Geometry: final body of the model. Coordinates: model frame, mm. A direction names the side the tool comes from. Round coordinates to 2 decimals unless told otherwise and drop trailing zeros. Order: outer loops, then holes, each group sorted by start corner. A loop starts at its lowest first (then second) coordinate and runs counter-clockwise, first axis right, second up. Notation, with made-up numbers: (21, 65.5) -> (66, 65.5) arc R18 ccw to (66, 69.5) -> close; hole circle Ø10 at (59, 82.25). An arc over 180 degrees is marked (long way). Put each result on its own line as item: value.
```python
from build123d import *

# Parameters (mm, degrees)
EXTRUDE_1_DEPTH      = 38
CUT_EXTRUDE_1_REACH  = 44.579
SKETCH_2_R           = 1.6
EXTRUDE_2_DEPTH      = 4.5
EXTRUDE_2_DEPTH_BACK = 10
SKETCH_3_R           = 1.15
CHAMFER_1_SIZE       = 0.2


with BuildPart() as part:
    # Эскиз1 → Бобышка-Вытянуть1 (new body)
    with BuildSketch(Plane.XY):
        with BuildLine():
            Line((-14.5, -3), (14.5, -3))
            Line((14.5, -3), (14.5, -1.148611647))
            ThreePointArc((14.5, -1.148611647), (14.150439729, -0.637384409), (13.547219321, -0.777637076))
            ThreePointArc((13.547219321, -0.777637076), (11.55, 0), (13.547219321, 0.777637076))
            ThreePointArc((13.547219321, 0.777637076), (13.692982689, 0.71288454), (13.839750373, 0.775327291))
            Line((13.839750373, 0.775327291), (15, 2))
            Line((15, 2), (15, 8.1))
            ThreePointArc((15, 8.1), (14.1, 9), (13.2, 8.1))
            Line((13.2, 8.1), (13.2, 2.602402736))
            ThreePointArc((13.2, 2.602402736), (11.012175957, 2.042975771), (10.05, 0))
            Line((10.05, 0), (9.55, 0))
            Line((9.55, 0), (9.55, 8.1))
            ThreePointArc((9.55, 8.1), (8.65, 9), (7.75, 8.1))
            Line((7.75, 8.1), (7.75, 0))
            Line((7.75, 0), (-7.75, 0))
            Line((-7.75, 0), (-7.75, 8.1))
            ThreePointArc((-7.75, 8.1), (-8.65, 9), (-9.55, 8.1))
            Line((-9.55, 8.1), (-9.55, 0))
            Line((-9.55, 0), (-10.05, 0))
            ThreePointArc((-10.05, 0), (-11.012175957, 2.042975771), (-13.2, 2.602402736))
            Line((-13.2, 2.602402736), (-13.2, 8.1))
            ThreePointArc((-13.2, 8.1), (-14.1, 9), (-15, 8.1))
            Line((-15, 8.1), (-15, 2))
            Line((-15, 2), (-13.839750373, 0.775327291))
            ThreePointArc((-13.839750373, 0.775327291), (-13.692982689, 0.71288454), (-13.547219321, 0.777637076))
            ThreePointArc((-13.547219321, 0.777637076), (-11.55, 0), (-13.547219321, -0.777637076))
            ThreePointArc((-13.547219321, -0.777637076), (-14.150439729, -0.637384409), (-14.5, -1.148611647))
            Line((-14.5, -1.148611647), (-14.5, -3))
        make_face()
    extrude(amount=EXTRUDE_1_DEPTH)

    # Эскиз2 → Вырез-Вытянуть1 (cut, up to next)
    with BuildSketch(Plane.XZ.offset(3), mode=Mode.PRIVATE) as cut_extrude_1_sk1:
        with Locations(Location((0, 18.3, 0), (0, 0, 270))):
            Circle(SKETCH_2_R)
    cut_extrude_1_tool1 = extrude(cut_extrude_1_sk1.sketch, amount=-CUT_EXTRUDE_1_REACH, mode=Mode.PRIVATE) & part.part
    add(cut_extrude_1_tool1.solids().sort_by_distance((0, -3, 18.3))[0], mode=Mode.SUBTRACT)

    # Эскиз3 → Бобышка-Вытянуть2 (add, two sides: drawn at the far end of the back side and taken through both)
    with BuildSketch(Plane(origin=(0, 0, 0), x_dir=(-1, 0, 0), z_dir=(0, 0, -1)).offset(-EXTRUDE_2_DEPTH_BACK)):
        with Locations((12.7, 0)):
            Circle(SKETCH_3_R)
        with Locations((-12.7, 0)):
            Circle(SKETCH_3_R)
    extrude(amount=EXTRUDE_2_DEPTH + EXTRUDE_2_DEPTH_BACK)

    # Фаска1
    chamfer_1_edges = [part.edges().sort_by_distance(p)[0] for p in [
        (-11.55, 0, -4.5),
        (13.85, 0, -4.5),
    ]]
    chamfer(chamfer_1_edges, length=CHAMFER_1_SIZE)


solid = part.part
```
1. Cut plane B-B on x = 0. Return loops of the section in (y, z), and give its area (3 significant figures).
Ans:
outline: (-3, 0) -> (0, 0) -> (0, 16.7) -> (-3, 16.7) -> close; (-3, 19.9) -> (0, 19.9) -> (0, 38) -> (-3, 38) -> close
area: 104 mm²
2. Cut plane A-A on y = 4.25. Return loops of the section in (x, z), and give its area (3 significant figures).
Ans:
outline: (-15, 0) -> (-13.2, 0) -> (-13.2, 38) -> (-15, 38) -> close; (-9.55, 0) -> (-7.75, 0) -> (-7.75, 38) -> (-9.55, 38) -> close; (7.75, 0) -> (9.55, 0) -> (9.55, 38) -> (7.75, 38) -> close; (13.2, 0) -> (15, 0) -> (15, 38) -> (13.2, 38) -> close
area: 274 mm²
3. Draft query along X for faces 1 (the face through (0, -1, 38)), 2 (the face through (-15, 5, 19)), 3 (the face through (7.75, 4, 19)), 4 (the face through (13, 0, 10)). Return one class per face: +X half, -X half, draft (parallel to the pull), parting line (faces both ways), or undercut.
Ans:
face 1: draft
face 2: -X half
face 3: undercut
face 4: undercut
4. Material intervals for probe 1 along X at (y, z) = (5, 20.5); probe 2 along Y at (x, z) = (12.7, 17.75); probe 3 along X at (y, z) = (-2.15, 18.3), sorted ascending.
Ans:
probe 1: -15 to -13.2, -9.55 to -7.75, 7.75 to 9.55, 13.2 to 15
probe 2: -3 to -1.15, 1.15 to 2.65
probe 3: -14.5 to -1.6, 1.6 to 14.5
5. Set-up query: faces 5 (the face through (13.2, 5, 19)), 6 (the face through (-14.43, 1.4, 18.73)), 7 (the face through (14.41, 1.38, 18.73)). Return all of +Z, -Z, +X, -X, +Y, -Y with unobstructed straight access to the full face (end or side cutting, diameter ignored); none if empty.
Ans:
face 5: +Z, -Z, +Y
face 6: +Z, -Z, -X
face 7: +Z, -Z, +X
6. Cut plane C-C on z = 7.5. Return loops of the section in (x, y), and give its area (3 significant figures).
Ans:
outline: (-15, 2) -> (-13.84, 0.78) arc R0.2 ccw to (-13.55, 0.78) arc R1.15 ccw to (-13.55, -0.78) arc R0.55 ccw to (-14.5, -1.15) -> (-14.5, -3) -> (14.5, -3) -> (14.5, -1.15) arc R0.55 ccw to (13.55, -0.78) arc R1.15 ccw to (13.55, 0.78) arc R0.2 ccw to (13.84, 0.78) -> (15, 2) -> (15, 8.1) arc R0.9 ccw to (13.2, 8.1) -> (13.2, 2.6) arc R2.65 ccw to (10.05, 0) -> (9.55, 0) -> (9.55, 8.1) arc R0.9 ccw to (7.75, 8.1) -> (7.75, 0) -> (-7.75, 0) -> (-7.75, 8.1) arc R0.9 ccw to (-9.55, 8.1) -> (-9.55, 0) -> (-10.05, 0) arc R2.65 ccw to (-13.2, 2.6) -> (-13.2, 8.1) arc R0.9 ccw to (-15, 8.1) -> close
area: 160 mm²
7. Cut plane D-D on x = -12.7. Return loops of the section in (y, z).
Ans:
outline: (-3, 0) -> (-1.15, 0) -> (-1.15, -4.3) -> (-0.95, -4.5) -> (0.95, -4.5) -> (1.15, -4.3) -> (1.15, 0) -> (2.65, 0) -> (2.65, 38) -> (1.15, 38) -> (1.15, 10) -> (-1.15, 10) -> (-1.15, 38) -> (-3, 38) -> close
8. Contact query for flat-ended pins moving along their axis: P1, Ø0.9, axis at y = -1.5, z = 18.5, coming from the +X side; P2, Ø2, axis at y = -2, z = 15, coming from the -X side; P3, Ø2, axis at x = 10.5, y = 7.5, coming from the -Z side. Output: stop coordinate, or through.
Ans:
P1: x = 14.5
P2: x = -14.5
P3: z = 0
